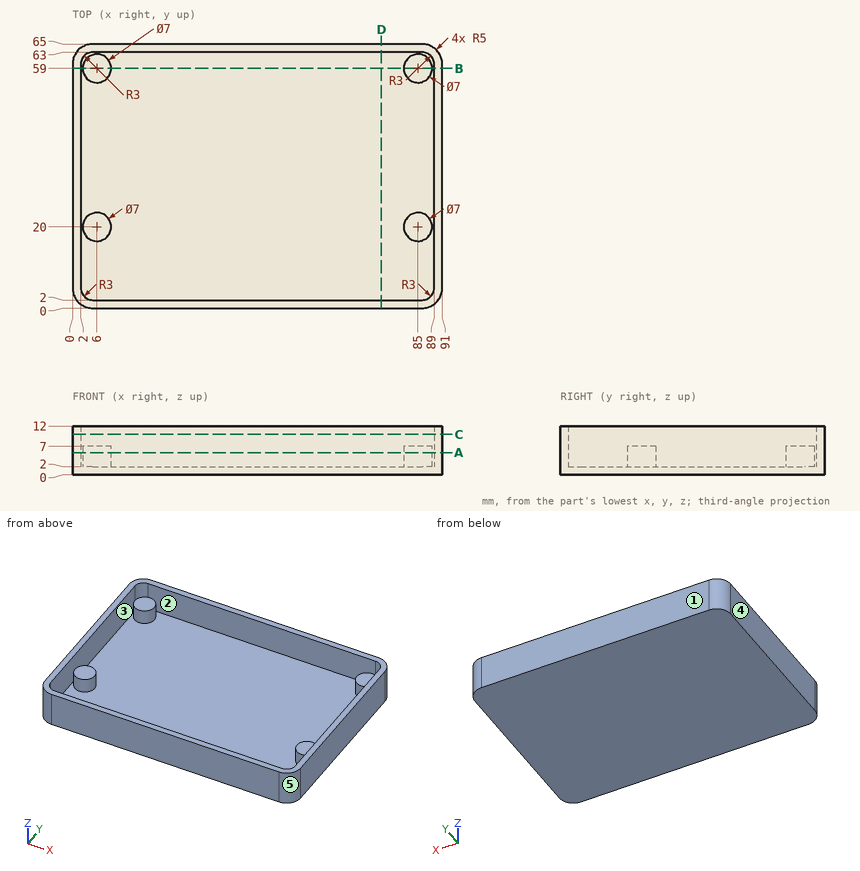
Here's the drawing with two shaded views (mm, measured from the low corner). I have some questions. A direction names the side the tool comes from. Round coordinates to 2 decimals unless told otherwise and drop trailing zeros. Loops run counter-clockwise (first coordinate to the right, second up) from the corner with the lowest first, then second, coordinate; pieces in that order, holes last. Notation, with made-up numbers: (-30.5, -20) - (-23.5, -20) arc R13 cw to (-23.5, 4) - close; hole circle Ø4 at (53.5, 31.25). An arc over 180 degrees is marked (long way). Write item = value, one per line.
1) On a 3-axis mill with a long thin cutter (end or side, diameter ignored), from which of +Z, -Z, +X, -X, +Y, -Y can I reach the whole of each face in a straight line? I mean the marked faces 1 and 2. Say none if no direction works.
Computed:
face_1 = +Z, -Z, +X, -X, +Y
face_2 = +Z
2) Imagine slicing it at C-C (z = 10). Please give me the cut outline in (x, y).
Computed:
outline = (0, 5) arc R5 ccw to (5, 0) - (86, 0) arc R5 ccw to (91, 5) - (91, 60) arc R5 ccw to (86, 65) - (5, 65) arc R5 ccw to (0, 60) - close; hole (2, 5) arc R3 ccw to (5, 2) - (86, 2) arc R3 ccw to (89, 5) - (89, 60) arc R3 ccw to (86, 63) - (5, 63) arc R3 ccw to (2, 60) - close
3) I need wall thicknesses on line 1 along Y through (x, z) = (73, 5.25); line 2 along X through (y, z) = (52.5, 8); line 3 along Y through (x, z) = (7.5, 2.5). Which ranges of each line are inside material? Lowest first, please. Write a range as from..to.
Computed:
line_1 = 0..2, 63..65
line_2 = 0..2, 89..91
line_3 = 0..2, 16.84..23.16, 55.84..62.16, 63..65
4) Imagine slicing it at D-D (x = 76). Please give me the cut outline in (y, z).
Computed:
outline = (0, 0) - (65, 0) - (65, 12) - (63, 12) - (63, 2) - (2, 2) - (2, 12) - (0, 12) - close
5) I'm going to push a flat-ended pin straight in: P1, Ø5.5, axis at x = 84, y = 60, coming from the +Z side. Where does the tip first touch, or does it pass through?
Computed:
P1 = 7
6) Imagine slicing it at B-B (y = 59). Please give me the cut outline in (x, z), and give its area (3 significant figures).
Computed:
outline = (0, 0) - (91, 0) - (91, 12) - (89, 12) - (89, 2) - (88.5, 2) - (88.5, 7) - (81.5, 7) - (81.5, 2) - (9.5, 2) - (9.5, 7) - (2.5, 7) - (2.5, 2) - (2, 2) - (2, 12) - (0, 12) - close
area = 292 mm2
7) Imagine slicing it at A-A (z = 5.5). Please give me the cut outline in (x, y).
Computed:
outline = (0, 5) arc R5 ccw to (5, 0) - (86, 0) arc R5 ccw to (91, 5) - (91, 60) arc R5 ccw to (86, 65) - (5, 65) arc R5 ccw to (0, 60) - close; circle Ø7 at (6, 20); circle Ø7 at (6, 59); circle Ø7 at (85, 20); circle Ø7 at (85, 59); hole (2, 5) arc R3 ccw to (5, 2) - (86, 2) arc R3 ccw to (89, 5) - (89, 60) arc R3 ccw to (86, 63) - (5, 63) arc R3 ccw to (2, 60) - close
8) If we mould it in two halves opening along X, with no side actions, what happens to the marked faces 3, 4 and 5? For each: pulls with the +X half, pulls with the -X half, needs draft (parallel to the pull), parting line crosses it, or undercut.
Computed:
face_3 = undercut
face_4 = pulls with the -X half
face_5 = pulls with the +X half
